Design review of the part built by this model. Coordinates are the model's own, in mm. Face numbers are marked on the shaded views. A direction names the side the tool comes from. Coordinates: 2 decimals unless noted, no trailing zeros. Write each loop counter-clockwise with the first axis right and the second up, starting at its lowest first coordinate (ties: lowest second). Pieces come first, ordered by that corner, then holes. Notation, with made-up numbers: (22.5, -12) - (50.5, -12) arc R19 cw to (50.5, 20) - close; hole circle Ø11 at (11.25, 85). An arc over 180 degrees is marked (long way). Answer as a JSON object with one key per item and string values.
Autodesk Inventor part; units mm, degrees
ref_plane "YZ Plane" through (0, 0, 0) normal (1, 0, 0) x (0, 1, 0)
ref_plane "XZ Plane" through (0, 0, 0) normal (0, 1, 0) x (-1, 0, 0)
ref_plane "XY Plane" through (0, 0, 0) normal (0, 0, 1) x (1, 0, 0)
sketch "Sketch1" plane through (0, 0, 0) normal (0, 1, 0) x (-1, 0, 0)
  line L0 (47.625, 47.625) -> (-47.625, 47.625)
  line L1 (-47.625, 47.625) -> (-47.625, -47.625)
  line L2 (-47.625, -47.625) -> (47.625, -47.625)
  line L3 (47.625, -47.625) -> (47.625, 47.625)
  line L4 (47.625, 47.625) -> (-47.625, -47.625) construction
  line L5 (-47.625, 47.625) -> (47.625, -47.625) construction
  point P0 (0, 0)
  dimension "d0" = 95.25
  dimension "d1" = 95.25
extrude "Extrusion1" add sketch "Sketch1" along normal blind 6.35
sketch "Sketch2" plane through (0, 6.35, 0) normal (0, 1, 0) x (1, 0, 0)
  line L0 (-12.7, -12.7) -> (12.7, -12.7)
  line L1 (12.7, -12.7) -> (12.7, 12.7)
  line L2 (12.7, 12.7) -> (-12.7, 12.7)
  line L3 (-12.7, 12.7) -> (-12.7, -12.7)
  line L4 (-12.7, -12.7) -> (12.7, 12.7) construction
  line L5 (12.7, -12.7) -> (-12.7, 12.7) construction
  line L6 (-9.525, -9.525) -> (9.525, -9.525)
  line L7 (9.525, -9.525) -> (9.525, 9.525)
  line L8 (9.525, 9.525) -> (-9.525, 9.525)
  line L9 (-9.525, 9.525) -> (-9.525, -9.525)
  line L10 (-9.525, -9.525) -> (9.525, 9.525) construction
  line L11 (9.525, -9.525) -> (-9.525, 9.525) construction
  line L12 (47.625, -47.625) -> (47.625, 47.625)
  line L13 (-47.625, -47.625) -> (47.625, -47.625)
  point P0 (0, 0)
  point P1 (0, 0)
  dimension "d4" = 25.4
  dimension "d5" = 25.4
  dimension "d6" = 3.175
  dimension "d7" = 3.175
  dimension "d8" = 34.925
  dimension "d14" = 34.925
extrude "Extrusion2" add sketch "Sketch2" along normal blind 119.9388
sketch "Sketch14" plane through (12.7, 6.35, 12.7) normal (1, 0, 0) x (0, 0, -1)
  line L0 (-34.925, -6.35) -> (60.325, -6.35)
  point P0 (12.7, -6.35)
  point P1 (12.7, 90.3478)
  dimension "d72" = 96.6978
hole "Hole6" at (12.7, 96.6978, 0) direction (-1, 0, 0) diameter 9.525 end through all
sketch "Sketch8" plane through (-12.7, 6.35, 12.7) normal (0, 0, 1) x (1, 0, 0)
  point P0 (12.7, 50.8)
sketch "Sketch9" plane through (-9.525, 6.35, -9.525) normal (0, 0, 1) x (1, 0, 0)
  point P0 (9.525, 50.8)
equation "\"d0\" = width"
equation "\"d1\" = length"
equation "\"d2\" = thickness"
equation "\"d9\" = heightOfPostAbovePlate"
equation "\"width\" = 95.25"
equation "\"length\" = 95.25"
equation "\"thickness\" = 6.35"
equation "\"totalHeight\" = 152.4"
equation "\"distanceFromFloorToBottomOfPan\" = 26.1112"
equation "\"thicknessOfPan\" = 3.175"
equation "\"heightOfPostAbovePlate\" = -thickness + totalHeight - distanceFromFloorToBottomOfPan"
properties part number "SupportPlateWithPostOnlyV01" material "Aluminum 6061"
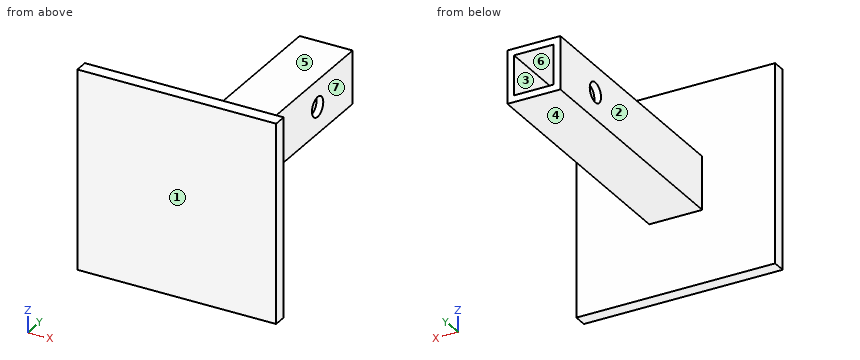
(1) To check wall thickness, follow line 1 (X direction, y = 104, z = 2) (3 decimals); line 2 (Y direction, x = 10, z = 0). State the ranges of each line that lie inside material, in increasing order. Write a range as from..to.
Solved:
{"line 1": "x = -12.7..-9.525, 9.525..12.7", "line 2": "y = 0..91.94, 101.46..126.29"}
(2) The part is to be moulded in two halves that separate along X. For the marked faces 5, 6 and 7, say which applies: pulls with the +X half, pulls with the -X half, needs draft (parallel to the pull), parting line crosses it, or undercut.
Solved:
{"face 5": "needs draft", "face 6": "undercut", "face 7": "pulls with the +X half"}
(3) Take a section at C-C, the plane x = 8. Write out the cut boundary in (y, z) (3 decimals).
Solved:
{"outline": "(0, -47.625) - (6.35, -47.625) - (6.35, -12.7) - (126.289, -12.7) - (126.289, -9.525) - (6.35, -9.525) - (6.35, 9.525) - (126.289, 9.525) - (126.289, 12.7) - (6.35, 12.7) - (6.35, 47.625) - (0, 47.625) - close"}
(4) Take a section at D-D, the plane z = 37. Write out the cut boundary in (x, y) (3 decimals), and give its area (3 significant figures).
Solved:
{"outline": "(-47.625, 0) - (47.625, 0) - (47.625, 6.35) - (-47.625, 6.35) - close", "area": "605 mm^2"}
(5) Take a section at B-B, the plane y = 20.5. Write out the cut boundary in (x, z) (3 decimals), and give its area (3 significant figures).
Solved:
{"outline": "(-12.7, -12.7) - (12.7, -12.7) - (12.7, 12.7) - (-12.7, 12.7) - close; hole (-9.525, -9.525) - (9.525, -9.525) - (9.525, 9.525) - (-9.525, 9.525) - close", "area": "282 mm^2"}
(6) Tool access review of the marked faces 1, 2, 3 and 4: name each direction out of +Z, -Z, +X, -X, +Y, -Y from which nothing blocks a thin tool from reaching the whole face with its end or side.
Solved:
{"face 1": "+Z, -Z, +X, -X, -Y", "face 2": "+Z, -Z, -X, +Y", "face 3": "+Y", "face 4": "-Z, +X, -X, +Y"}
(7) Take a section at A-A, the plane z = 0. Write out the cut boundary in (x, y) (3 decimals), and give its area (3 significant figures).
Solved:
{"outline": "(-47.625, 0) - (47.625, 0) - (47.625, 6.35) - (12.7, 6.35) - (12.7, 91.935) - (9.525, 91.935) - (9.525, 6.35) - (-9.525, 6.35) - (-9.525, 91.935) - (-12.7, 91.935) - (-12.7, 6.35) - (-47.625, 6.35) - close; (-12.7, 101.46) - (-9.525, 101.46) - (-9.525, 126.289) - (-12.7, 126.289) - close; (9.525, 101.46) - (12.7, 101.46) - (12.7, 126.289) - (9.525, 126.289) - close", "area": "1,310 mm^2"}
(8) For pin 1 (9.5 mm diameter, centred on x = 0.5, y = 82, fed in from +Z); pin 2 (15 mm diameter, centred on y = 94.5, z = 3, fed in from +X); pin 3 (5.5 mm diameter, centred on y = 95, z = -2.5, fed in from -X), all flat-tipped, find the tip position at first contact; note any pin that passes through.
Solved:
{"pin 1": "stops at z = 12.7", "pin 2": "stops at x = 12.7", "pin 3": "stops at x = -12.7"}
